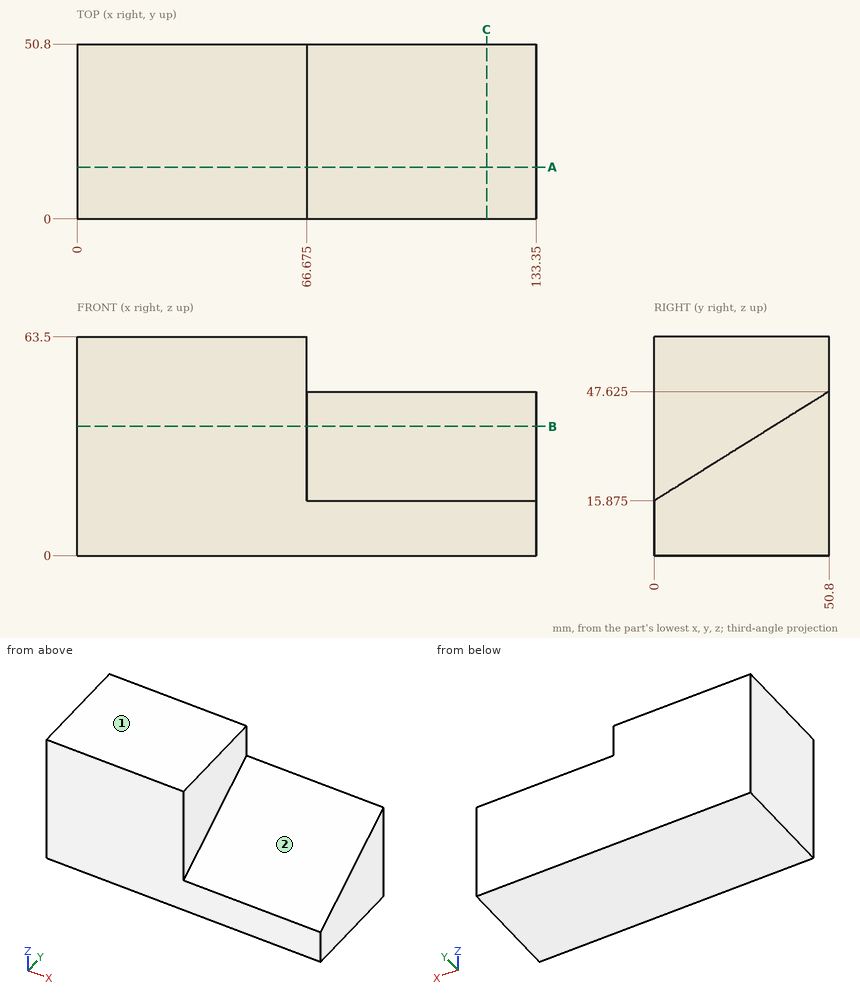
Print and shaded views of the part. All mm, measured from the part's lowest x, y and z. A direction names the side the tool comes from. Give positions to 0.01 mm unless a question says otherwise; leave off trailing zeros. Write each loop counter-clockwise with the first axis right and the second up, starting at its lowest first coordinate (ties: lowest second). Pieces come first, ordered by that corner, then holes. Notation, with made-up numbers: (32, 22.5) -> (67, 22.5) arc R20 cw to (67, 33.5) -> close; hole circle Ø1 at (-8.5, 30). An arc over 180 degrees is marked (long way). Write item = value, one per line.
(1) Flat gauge pin, fed straight in: P1, Ø1, axis at x = 84.5, y = 13.5, coming from the +Z side (3 decimals). Where does the tip first touch, or does it go through?
Determined:
P1 = 24.625
(2) Probe line 1 along X through (y, z) = (12, 27.5) (3 decimals); line 2 along Y through (x, z) = (121, 34); line 3 along Z through (x, y) = (85, 34) (3 decimals). List the from-to ranges inside material, lowest first.
Determined:
line_1 = 0 to 66.675
line_2 = 29 to 50.8
line_3 = 0 to 37.125
(3) Slice it at B-B, the plane z = 37.5. Give the cut face in (x, y) (3 decimals).
Determined:
outline = (0, 0) -> (66.675, 0) -> (66.675, 34.6) -> (133.35, 34.6) -> (133.35, 50.8) -> (0, 50.8) -> close
(4) Slice it at A-A, the plane y = 15. Give the cut face in (x, z) (3 decimals), then the cut area to 3 significant figures.
Determined:
outline = (0, 0) -> (133.35, 0) -> (133.35, 25.25) -> (66.675, 25.25) -> (66.675, 63.5) -> (0, 63.5) -> close
area = 5,920 mm2
(5) Tool access for the marked faces 1 and 2: list every direction of +Z, -Z, +X, -X, +Y, -Y with a clear straight run to the whole face (end or side of a thin tool).
Determined:
face_1 = +Z, +X, -X, +Y, -Y
face_2 = +Z, +X, -Y
(6) Slice it at C-C, the plane x = 119. Give the cut face in (y, z) (3 decimals).
Determined:
outline = (0, 0) -> (50.8, 0) -> (50.8, 47.625) -> (0, 15.875) -> close
